Verification items for this drawing (mm, ordinates from the low corner). A direction names the side the tool comes from. Coordinates: 2 decimals unless noted, no trailing zeros. Order: outer loops, then holes, each group sorted by start corner. A loop starts at its lowest first (then second) coordinate and runs counter-clockwise, first axis right, second up.
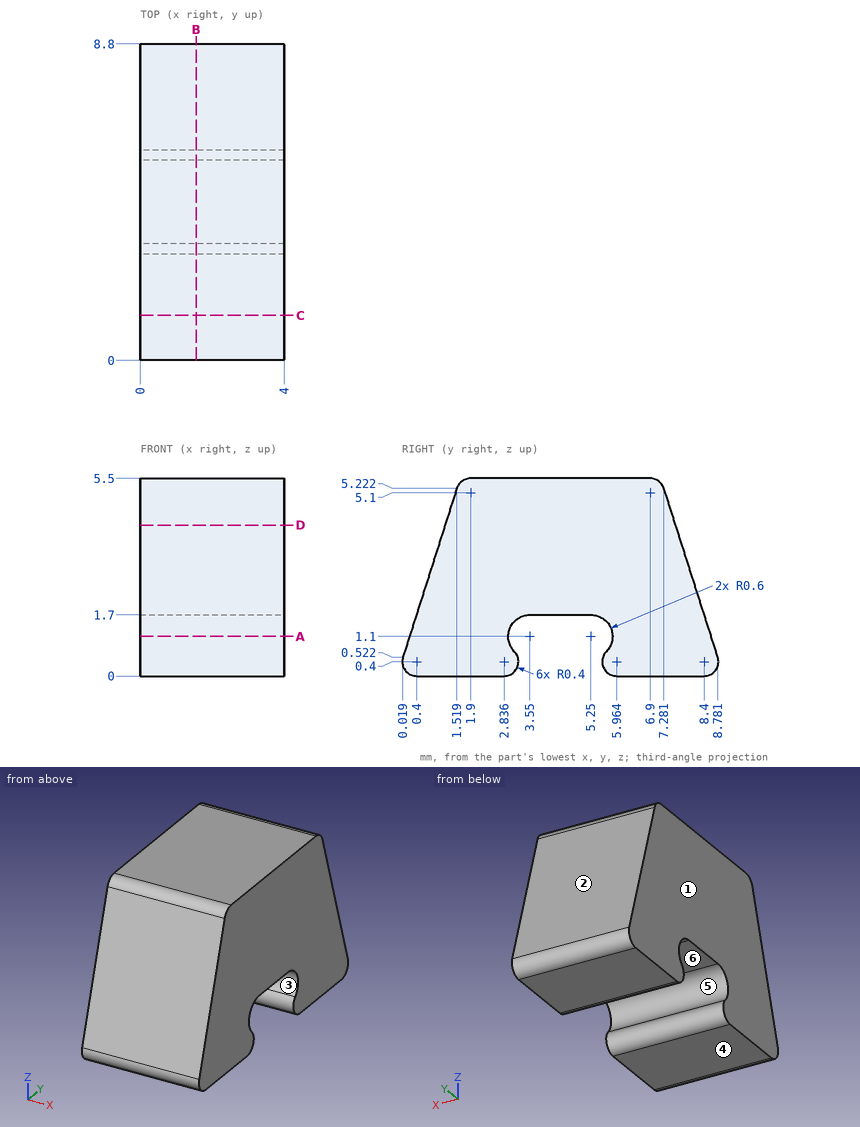
(1) Go/stop test with flat-tipped pins: P1, Ø1.4, axis at x = 1.5, y = 4.5, coming from the -Z side; P2, Ø1.5, axis at x = 3, z = 4, coming from the +Y side. Record where each tip stops, or that it passes through.
Filled in:
P1: stops at z = 1.7
P2: stops at y = 7.91
(2) Cross-section at C-C (y = 1.25). Enter the section's corners in (x, z), and give its area (3 significant figures).
Filled in:
outline: (0, 0) - (4, 0) - (4, 4.38) - (0, 4.38) - close
area: 17.5 mm2
(3) Cross-section at A-A (z = 1.1). Enter the section's corners in (x, y), and give its area (3 significant figures).
Filled in:
outline: (0, 0.2) - (4, 0.2) - (4, 2.95) - (0, 2.95) - close; (0, 5.85) - (4, 5.85) - (4, 8.6) - (0, 8.6) - close
area: 22.0 mm2
(4) Cross-section at B-B (x = 1.55). Enter the section's corners in (y, z).
Filled in:
outline: (0.02, 0.52) arc R0.4 ccw to (0.4, 0) - (2.84, 0) arc R0.4 ccw to (3.12, 0.68) arc R0.6 cw to (3.55, 1.7) - (5.25, 1.7) arc R0.6 cw to (5.68, 0.68) arc R0.4 ccw to (5.96, 0) - (8.4, 0) arc R0.4 ccw to (8.78, 0.52) - (7.28, 5.22) arc R0.4 ccw to (6.9, 5.5) - (1.9, 5.5) arc R0.4 ccw to (1.52, 5.22) - close
(5) Release check for a two-part mould opening along Y. For the marked faces 1, 2 and 3 record: +Y half, -Y half, draft (parallel to the pull), parting line (faces both ways), or undercut.
Filled in:
face 1: draft
face 2: +Y half
face 3: undercut
(6) Thickness scan on probe 1 along Y at (x, z) = (2.25, 0.35); probe 2 along Y at (x, z) = (3, 0.2) (1 decimal); probe 3 along Z at (x, y) = (1.1, 3.5). Record the ranges inside material, lowest first.
Filled in:
probe 1: y = 0 to 3.23, 5.57 to 8.8
probe 2: y = 0.1 to 3.2, 5.6 to 8.7
probe 3: z = 1.7 to 5.5
(7) Tool access check on the marked faces 4, 5 and 6. Record the directions out of +Z, -Z, +X, -X, +Y, -Y that give a thin tool (end or side, any length) a straight path to the whole face; none if there is none.
Filled in:
face 4: -Z, +X, -X, +Y, -Y
face 5: +X, -X
face 6: -Z, +X, -X
(8) Cross-section at D-D (z = 4.2). Enter the section's corners in (x, y).
Filled in:
outline: (0, 1.19) - (4, 1.19) - (4, 7.61) - (0, 7.61) - close
